Work out the finished part from the listing and answer in its coordinate system (mm). A direction names the side the tool comes from. Coordinates: 2 decimals unless noted, no trailing zeros. Order: outer loops, then holes, each group sorted by start corner. A loop starts at its lowest first (then second) coordinate and runs counter-clockwise, first axis right, second up. Notation, with made-up numbers: M -26.75,-1 L 14.25,-1 A16 cw 14.25,5 Z; hole C 32,24.5 d3. An arc over 180 degrees is marked long. Answer in a Markdown table with one row per item. Add a question column.
Item 1: Flat-ended cylindrical pins translate along their axes: pin 1 Ø4 at (x, z) = (12.85, 5) entering from +Y; pin 2 Ø3 at (x, y) = (16.5, 3.5) entering from +Z; pin 3 Ø1 at (x, y) = (12.5, 4.5) entering from +Z; pin 4 Ø3.5 at (y, z) = (1, 4) entering from +X. Find the tip coordinate at first contact, or state that the pin passes through.
Item 2: The part is cut by section B-B (y = 2). Write down the section's boundary in (x, z).
Item 3: The part is cut by section C-C (x = 3). Write down the section's boundary in (y, z), then the cut area to 3 significant figures.
Item 4: The part is cut by section A-A (z = 5). Write down the section's boundary in (x, y), then the cut area to 3 significant figures.
Item 5: Consider line 1 (X direction, y = 1.8, z = 5); line 2 (Y direction, x = 3, z = 0.6); line 3 (Z direction, x = 20.85, y = 2.05). Determine where each line is inside the solid, lowest interval first. Write a range as from..to.
Item 6: The part is cut by section D-D (y = 4.5). Write down the section's boundary in (x, z).
Item 7: Which of the six approach directions +Z, -Z, +X, -X, +Y, -Y give full straight-line access (tool end or side, diameter ignored) to faces 4 (the face through (24.85, 1, 5)), 5 (the face through (8.85, 1, 5)), 6 (the face through (17, 3, 5))?
Item 8: The mould has two halves that part along X. Classify faces 1 (the face through (0, 3, 1)), 2 (the face through (29.05, 3.22, 0.99)), 3 (the face through (17, 0, 3)): released by +X, released by -X, zero draft, split by the parting line, or undercut.
from build123d import *

# Parameters (mm, degrees)
SKETCH1_W           = 33.7
SKETCH1_H           = 6.3
SKETCH1_R           = 1.65
BOSS_EXTRUDE1_DEPTH = 2
SKETCH2_W           = 16
SKETCH2_H           = 3
BOSS_EXTRUDE2_DEPTH = 6
SKETCH3_R           = 1.65
CUT_EXTRUDE1_DEPTH  = 6


with BuildPart() as part:
    # Sketch1 → Boss-Extrude1 (new body)
    with BuildSketch(Plane.XY):
        with Locations((16.85, 3.15)):
            Rectangle(SKETCH1_W, SKETCH1_H)
        with Locations((3, 3.15)):
            Circle(SKETCH1_R, mode=Mode.SUBTRACT)
        with Locations((30.7, 3.15)):
            Circle(SKETCH1_R, mode=Mode.SUBTRACT)
    extrude(amount=BOSS_EXTRUDE1_DEPTH)

    # Sketch2 → Boss-Extrude2 (add)
    with BuildSketch(Plane.XY.offset(2)):
        with Locations((16.85, 1.5)):
            Rectangle(SKETCH2_W, SKETCH2_H)
    extrude(amount=BOSS_EXTRUDE2_DEPTH)

    # Sketch3 → Cut-Extrude1 (cut)
    with BuildSketch(Plane(origin=(0, 3, 0), x_dir=(1, 0, 0), z_dir=(0, 1, 0))):
        with Locations((12.85, -5)):
            Circle(SKETCH3_R)
        with Locations((20.85, -5)):
            Circle(SKETCH3_R)
    extrude(amount=-CUT_EXTRUDE1_DEPTH, mode=Mode.SUBTRACT)


solid = part.part
Reply:
| question | item | result |
|---|---|---|
| 1 | pin 1 | stops at y = 3 |
| 1 | pin 2 | stops at z = 8 |
| 1 | pin 3 | stops at z = 2 |
| 1 | pin 4 | stops at x = 24.85 |
| 2 | outline | M 0,0 L 1.82,0 L 1.82,2 L 0,2 Z; M 4.18,0 L 29.52,0 L 29.52,2 L 24.85,2 L 24.85,8 L 8.85,8 L 8.85,2 L 4.18,2 Z; M 31.88,0 L 33.7,0 L 33.7,2 L 31.88,2 Z; hole C 12.85,5 d3.3; hole C 20.85,5 d3.3 |
| 3 | outline | M 0,0 L 1.5,0 L 1.5,2 L 0,2 Z; M 4.8,0 L 6.3,0 L 6.3,2 L 4.8,2 Z |
| 3 | area | 6.00 mm2 |
| 4 | outline | M 8.85,0 L 11.2,0 L 11.2,3 L 8.85,3 Z; M 14.5,0 L 19.2,0 L 19.2,3 L 14.5,3 Z; M 22.5,0 L 24.85,0 L 24.85,3 L 22.5,3 Z |
| 4 | area | 28.2 mm2 |
| 5 | line 1 | x = 8.85..11.2, 14.5..19.2, 22.5..24.85 |
| 5 | line 2 | y = 0..1.5, 4.8..6.3 |
| 5 | line 3 | z = 0..3.35, 6.65..8 |
| 6 | outline | M 0,0 L 2.05,0 L 2.05,2 L 0,2 Z; M 3.95,0 L 29.75,0 L 29.75,2 L 3.95,2 Z; M 31.65,0 L 33.7,0 L 33.7,2 L 31.65,2 Z |
| 7 | face 4 | +Z, +X, +Y, -Y |
| 7 | face 5 | +Z, -X, +Y, -Y |
| 7 | face 6 | +Z, +X, -X, +Y |
| 8 | face 1 | released by -X |
| 8 | face 2 | undercut |
| 8 | face 3 | zero draft |
